Geometry check sheet. Reference: the model listing, model coordinates, mm. A direction names the side the tool comes from. Give positions to 0.01 mm unless a question says otherwise; leave off trailing zeros. Loops run counter-clockwise (first coordinate to the right, second up) from the corner with the lowest first, then second, coordinate; pieces in that order, holes last. Notation, with made-up numbers: (-16.75, -21.75) -> (-8.75, -21.75) arc R19 ccw to (-8.75, 9.25) -> close; hole circle Ø11 at (85.25, 17.5). An arc over 180 degrees is marked (long way). One line per item, written item: value. Start each with the question number.
(1) Draft check along Z on faces 3 (the face through (4, 19, 0)), 4 (the face through (304.8, 19, 15)), 5 (the face through (4, 26, 25.4)), 6 (the face through (4, 10, 38.1)). Enter one of: pulls with the +Z half, pulls with the -Z half, needs draft (parallel to the pull), parting line crosses it, or undercut.
(2) Scan lines: line 1 along X through (y, z) = (11, 12); line 2 along X through (y, z) = (35, 2.5) (3 decimals); line 3 along Z through (x, y) = (151.5, 34). Record each from-to range of solid material in increasing order. Write a range as from..to.
(3) Tool access check on faces 1 (the face through (300, 38.1, 13)), 2 (the face through (272, 33.338, 13)). Record the directions out of +Z, -Z, +X, -X, +Y, -Y that give a thin tool (end or side, any length) a straight path to the whole face; none if there is none.
(4) Sectioned sample at A-A, the plane x = -123. Record the cut outline in (y, z), then the cut area to 3 significant figures.
(5) Gauge pin test, flat ends, axial feed: pin 1 Ø3 at (x, y) = (-141.5, 9) entering from -Z; pin 2 Ø1 at (x, y) = (-129, 23.5) entering from +Z. Record the tip position at first contact, or that the pin passes through.
from build123d import *

# Parameters (mm, degrees)
F1_DEPTH      = 304.8
F1_DEPTH_BACK = 304.8
F2_W          = 38.1
F2_H          = 4.7625
F3_DEPTH      = 25.401
F5_D          = 7.9375
F7_DEPTH      = 609.6


with BuildPart() as f1:
    # F0 (on Right) → F1 (new body, two sides)
    with BuildSketch(Plane.YZ) as f1_sk:
        Polygon((0, 38.1), (0, 0), (38.1, 0), (38.1, 25.4), (12.7, 25.4), (12.7, 38.1), align=None)
    extrude(amount=F1_DEPTH)
    extrude(f1_sk.sketch, amount=-F1_DEPTH_BACK)

    # F2 (on face) → F3 (cut, through all)
    with BuildSketch(Plane.XY.offset(25.4)):
        with Locations((-50.8, 35.71875)):
            Rectangle(F2_W, F2_H)
        with Locations((276.225, 35.71875)):
            Rectangle(F2_W, F2_H)
    extrude(amount=-F3_DEPTH, mode=Mode.SUBTRACT)

    # F5 (through all)
    with Locations(Plane(origin=(0, 33.3375, 0), x_dir=(-1, 0, 0), z_dir=(0, 1, 0))):
        with Locations((-276.225, 12.7), (50.8, 12.7)):
            Hole(F5_D / 2)

    # F6 (on face) → F7 (join, through all)
    with BuildSketch(Plane.YZ.offset(304.8)):
        Polygon((20.032348, 38.1), (12.7, 38.1), (12.7, 25.4), align=None)
    extrude(amount=-F7_DEPTH)


solid = f1.part
Calculated:
1. face 3: pulls with the -Z half
1. face 4: needs draft
1. face 5: undercut
1. face 6: pulls with the +Z half
2. line 1: x = -304.8..-54.71, -46.89..272.32, 280.13..304.8
2. line 2: x = -304.8..-69.85, -31.75..257.175, 295.275..304.8
2. line 3: z = 0..25.4
3. face 1: +Z, -Z, +X, -X, +Y
3. face 2: +Z, -Z, +Y
4. outline: (0, 0) -> (38.1, 0) -> (38.1, 25.4) -> (12.7, 25.4) -> (20.03, 38.1) -> (0, 38.1) -> close
4. area: 1,180 mm2
5. pin 1: stops at z = 0
5. pin 2: stops at z = 25.4
